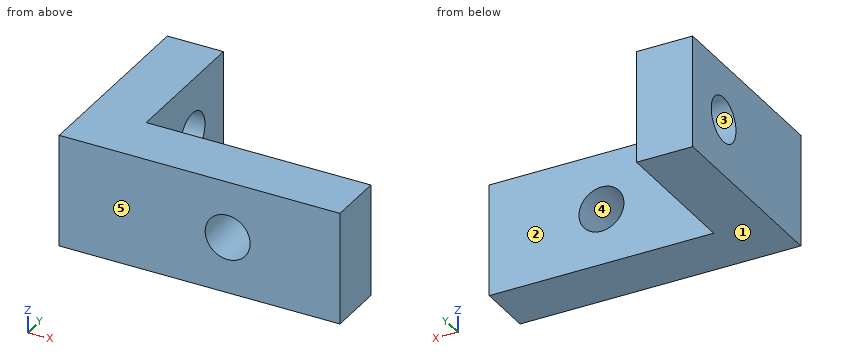
```python
from build123d import *

# Parameters (mm, degrees)
BOSS_EXTRUDE2_DEPTH = 5.08
SKETCH3_R           = 1.016
CUT_EXTRUDE1_DEPTH  = 25.4
SKETCH4_R           = 1.016
CUT_EXTRUDE2_DEPTH  = 2.54


with BuildPart() as part:
    # Sketch1 → Boss-Extrude2 (new body)
    with BuildSketch(Plane.XY):
        Polygon((-15.917333333, -20.997333333), (-15.917333333, -29.887333333), (-3.217333333, -29.887333333), (-3.217333333, -27.347333333), (-13.377333333, -27.347333333), (-13.377333333, -20.997333333), align=None)
    extrude(amount=BOSS_EXTRUDE2_DEPTH)

    # Sketch3 → Cut-Extrude1 (cut)
    with BuildSketch(Plane(origin=(0, -27.347333333, 0), x_dir=(1, 0, 0), z_dir=(0, 1, 0))):
        with Locations((-8.297333333, -2.54)):
            Circle(SKETCH3_R)
    extrude(amount=-CUT_EXTRUDE1_DEPTH, mode=Mode.SUBTRACT)

    # Sketch4 → Cut-Extrude2 (cut)
    with BuildSketch(Plane.ZY.offset(15.917333333)):
        with Locations((2.54, -23.537333333)):
            Circle(SKETCH4_R)
    extrude(amount=-CUT_EXTRUDE2_DEPTH, mode=Mode.SUBTRACT)


solid = part.part
```
Input: part model. Units: mm. Frame: model coordinates. Face numbers are marked on the shaded views. A direction names the side the tool comes from. Round coordinates to 2 decimals unless told otherwise and drop trailing zeros. Loops run counter-clockwise (first coordinate to the right, second up) from the corner with the lowest first, then second, coordinate; pieces in that order, holes last. Notation, with made-up numbers: (14.5, -19.75) - (28.5, -19.75) arc R21 cw to (28.5, 7.25) - close; hole circle Ø11 at (7.25, 78.5). An arc over 180 degrees is marked (long way). One line per item, written item: value. Start each with the question number.
(1) Draft query along Y for the marked faces 3, 4 and 5. Return one class per face: +Y half, -Y half, draft (parallel to the pull), parting line (faces both ways), or undercut.
(2) Section C-C, the plane x = -8. Return loops of the section in (y, z), plus the area to 3 significant figures.
(3) Section B-B, the plane y = -24. Return loops of the section in (x, z).
(4) Section D-D, the plane x = -13.75. Return loops of the section in (y, z).
(5) Access query for the marked faces 1 and 2. Directions: +Z, -Z, +X, -X, +Y, -Y. A direction counts if a zero-diameter tool reaches every point of the face in a straight line with its end or side. Return the directions, or none.
(6) Section A-A, the plane z = 2.54. Return loops of the section in (x, y).
(7) Contact query for flat-ended pins moving along their axis: P1, Ø2.5, axis at y = -24.5, z = 3, coming from the +X side; P2, Ø2.5, axis at x = -8.3, z = 2.54, coming from the -Y side; P3, Ø1.2, axis at y = -23.54, z = 2.54, coming from the -X side. Output: stop coordinate, or through.
(8) Ray query, line 1 (Y direction, x = -14.3, z = 2.54); line 2 (X direction, y = -28.4, z = 2.54); line 3 (Y direction, x = -10.5, z = 2.9). Return the intervals inside material, ascending. Write a range as [from, to].
Results below:
1. face 3: undercut
1. face 4: draft
1. face 5: -Y half
2. outline: (-29.89, 0) - (-27.35, 0) - (-27.35, 1.57) - (-29.89, 1.57) - close; (-29.89, 3.51) - (-27.35, 3.51) - (-27.35, 5.08) - (-29.89, 5.08) - close
2. area: 7.97 mm^2
3. outline: (-15.92, 0) - (-13.38, 0) - (-13.38, 1.64) - (-15.92, 1.64) - close; (-15.92, 3.44) - (-13.38, 3.44) - (-13.38, 5.08) - (-15.92, 5.08) - close
4. outline: (-29.89, 0) - (-21, 0) - (-21, 5.08) - (-29.89, 5.08) - close; hole circle Ø2.03 at (-23.54, 2.54)
5. face 1: -Z, +X, -X, +Y, -Y
5. face 2: +Z, -Z, +X, +Y
6. outline: (-15.92, -29.89) - (-9.31, -29.89) - (-9.31, -27.35) - (-13.38, -27.35) - (-13.38, -24.55) - (-15.92, -24.55) - close; (-15.92, -22.52) - (-13.38, -22.52) - (-13.38, -21) - (-15.92, -21) - close; (-7.28, -29.89) - (-3.22, -29.89) - (-3.22, -27.35) - (-7.28, -27.35) - close
7. P1: x = -13.38
7. P2: y = -29.89
7. P3: through
8. line 1: [-29.89, -24.55], [-22.52, -21]
8. line 2: [-15.92, -9.31], [-7.28, -3.22]
8. line 3: [-29.89, -27.35]
